Geometry check sheet. Reference: the model listing, model coordinates, mm. Face numbers are marked on the shaded views. A direction names the side the tool comes from. Round coordinates to 2 decimals unless told otherwise and drop trailing zeros. Write each loop counter-clockwise with the first axis right and the second up, starting at its lowest first coordinate (ties: lowest second). Pieces come first, ordered by that corner, then holes. Notation, with made-up numbers: (7.25, 4) -> (37.25, 4) arc R13 ccw to (37.25, 8) -> close; hole circle Ø11 at (-13, 53). An arc over 180 degrees is marked (long way). One line per question, with ' | ' between items.
```python
from build123d import *

# Parameters (mm, degrees)
BOSS_EXTRUDE1_DEPTH = 482.6
BOSS_EXTRUDE2_REACH = 1843.631
CUT_EXTRUDE2_DEPTH  = 2063.411181118
SKETCH9_R           = 114.3
CUT_EXTRUDE3_DEPTH  = 1996.153427684


with BuildPart() as part:
    # Sketch1 → Boss-Extrude1 (new, symmetric)
    with BuildSketch(Plane.XY):
        with BuildLine():
            Line((-914.4, 0), (-685.8, 0))
            ThreePointArc((-685.8, 0), (0, 685.8), (685.8, 0))
            Line((685.8, 0), (914.4, 0))
            ThreePointArc((914.4, 0), (0, 914.4), (-914.4, 0))
        make_face()
    extrude(amount=BOSS_EXTRUDE1_DEPTH, both=True)

    # Boss-Extrude2: up to this face of the body (flat: up to its plane)
    boss_extrude2_end = Plane(part.part.faces().sort_by_distance((-800.1, 0, 0))[0])
    # Sketch7 → Boss-Extrude2 (add, up to the picked face)
    with BuildSketch(Plane(origin=(0, 1524, 0), x_dir=(-1, 0, 0), z_dir=(0, -1, 0)), mode=Mode.PRIVATE) as boss_extrude2_sk1:
        with BuildLine():
            Line((965.2, -228.6), (-965.2, -228.6))
            ThreePointArc((-965.2, -228.6), (-1193.8, 0), (-965.2, 228.6))
            Line((-965.2, 228.6), (965.2, 228.6))
            ThreePointArc((965.2, 228.6), (1193.8, 0), (965.2, -228.6))
        make_face()
    boss_extrude2_tool1 = split(extrude(boss_extrude2_sk1.sketch, amount=BOSS_EXTRUDE2_REACH, mode=Mode.PRIVATE), bisect_by=boss_extrude2_end, keep=Keep.BOTH, mode=Mode.PRIVATE)
    add(boss_extrude2_tool1.solids().sort_by(Axis((0, 1524, 0), (0, -1, 0)))[0])

    # Sketch8 → Cut-Extrude2 (cut, through all)
    with BuildSketch(Plane.XY.offset(228.6)):
        with BuildLine():
            Line((-685.8, 0), (685.8, 0))
            ThreePointArc((685.8, 0), (0, 685.8), (-685.8, 0))
        make_face()
    extrude(amount=-CUT_EXTRUDE2_DEPTH, mode=Mode.SUBTRACT)

    # Sketch9 → Cut-Extrude3 (cut, through all)
    with BuildSketch(Plane.XZ):
        with Locations(Location((-965.2, 0, 0), (0, 0, 270))):
            Circle(SKETCH9_R)
        with Locations(Location((965.2, 0, 0), (0, 0, 270))):
            Circle(SKETCH9_R)
    extrude(amount=-CUT_EXTRUDE3_DEPTH, mode=Mode.SUBTRACT)


solid = part.part
```
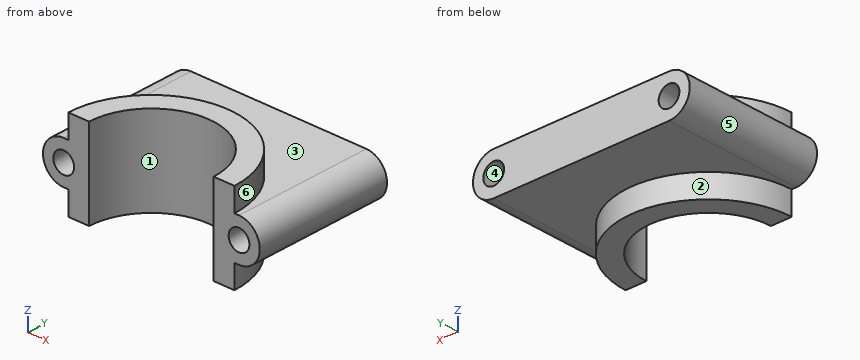
(1) Access from +Z, -Z, +X, -X, +Y, -Y to the whole of each face (thin tool, end or side, straight path). Record for the marked faces 1 and 2.
Resolved:
face 1: +Z, -Z, -Y | face 2: -Z, +Y
(2) Sectioned sample at C-C on x = 0. Record the cut outline in (y, z).
Resolved:
outline: (685.8, -482.6) -> (914.4, -482.6) -> (914.4, -228.6) -> (1524, -228.6) -> (1524, 228.6) -> (914.4, 228.6) -> (914.4, 482.6) -> (685.8, 482.6) -> close
(3) Sectioned sample at D-D on y = 1129. Record the cut outline in (x, z), then the cut area to 3 significant figures.
Resolved:
outline: (-965.2, -228.6) -> (965.2, -228.6) arc R228.6 ccw to (965.2, 228.6) -> (-965.2, 228.6) arc R228.6 ccw to start; hole circle Ø228.6 at (-965.2, 0); hole circle Ø228.6 at (965.2, 0) | area: 965,000 mm2
(4) Sectioned sample at A-A on z = 0. Record the cut outline in (x, y), then the cut area to 3 significant figures.
Resolved:
outline: (-1193.8, 0) -> (-1079.5, 0) -> (-1079.5, 1524) -> (-1193.8, 1524) -> close; (-850.9, 0) -> (-685.8, 0) arc R685.8 cw to (685.8, 0) -> (850.9, 0) -> (850.9, 1524) -> (-850.9, 1524) -> close; (1079.5, 0) -> (1193.8, 0) -> (1193.8, 1524) -> (1079.5, 1524) -> close | area: 2,200,000 mm2
(5) Draft check along Z on the marked faces 3, 4, 5 and 6. Enter one of: +Z half, -Z half, draft (parallel to the pull), parting line (faces both ways), or undercut.
Resolved:
face 3: +Z half | face 4: undercut | face 5: parting line | face 6: draft
(6) Sectioned sample at B-B on y = 202.5. Record the cut outline in (x, z), then the cut area to 3 significant figures.
Resolved:
outline: (-965.2, -228.6) -> (-891.7, -228.6) -> (-891.7, -482.6) -> (-655.22, -482.6) -> (-655.22, 482.6) -> (-891.7, 482.6) -> (-891.7, 228.6) -> (-965.2, 228.6) arc R228.6 ccw to start; (655.22, -482.6) -> (891.7, -482.6) -> (891.7, -228.6) -> (965.2, -228.6) arc R228.6 ccw to (965.2, 228.6) -> (891.7, 228.6) -> (891.7, 482.6) -> (655.22, 482.6) -> close; hole circle Ø228.6 at (-965.2, 0); hole circle Ø228.6 at (965.2, 0) | area: 606,000 mm2
(7) Go/stop test with flat-tipped pins: pin 1 (8 mm diameter, centred on x = -291.5, z = 290, fed in from -Y); pin 2 (6 mm diameter, centred on x = 436.5, y = 911, fed in from +Z); pin 3 (4 mm diameter, centred on y = 298.5, z = 292.5, fed in from -X). Record where each tip stops, or that it passes through.
Resolved:
pin 1: stops at y = 618.87 | pin 2: stops at z = 228.6 | pin 3: stops at x = -864.99
(8) Material ranges on line 1 (X direction, y = 725, z = 0); line 2 (X direction, y = 474, z = -43.5); line 3 (X direction, y = 491, z = 0), recorded low to high.
Resolved:
line 1: x = -1193.8 to -1079.5, -850.9 to 850.9, 1079.5 to 1193.8 | line 2: x = -1189.62 to -1070.9, -859.5 to -495.63, 495.63 to 859.5, 1070.9 to 1189.62 | line 3: x = -1193.8 to -1079.5, -850.9 to -478.79, 478.79 to 850.9, 1079.5 to 1193.8
